from build123d import *

# Parameters (mm, degrees)
F1_DEPTH = 500
F2_R     = 2
F3_R     = 1.5
F4_R     = 1.5


with BuildPart() as f1:
    # F0 (on Front) → F1 (new body)
    with BuildSketch(Plane.XZ):
        Polygon((-12.5, 18.558511), (-22.5, 18.558511), (-22.5, 3.558511), (22.5, 3.558511), (22.5, 18.558511), (12.5, 18.558511), (12.5, 16.058511), (20, 16.058511), (20, 6.058511), (-20, 6.058511), (-20, 16.058511), (-12.5, 16.058511), align=None)
    extrude(amount=F1_DEPTH)

    # F2
    f2_edges = [f1.edges().sort_by_distance(p)[0] for p in [
        (22.5, -250, 18.558511),
        (-22.5, -250, 18.558511),
        (-22.5, -250, 3.558511),
        (22.5, -250, 3.558511),
    ]]
    fillet(f2_edges, radius=F2_R)

    # F3
    f3_edges = [f1.edges().sort_by_distance(p)[0] for p in [
        (20, -250, 16.058511),
        (-20, -250, 16.058511),
    ]]
    fillet(f3_edges, radius=F3_R)

    # F4
    f4_edges = [f1.edges().sort_by_distance(p)[0] for p in [
        (-20, -250, 6.058511),
        (20, -250, 6.058511),
    ]]
    fillet(f4_edges, radius=F4_R)


solid = f1.part
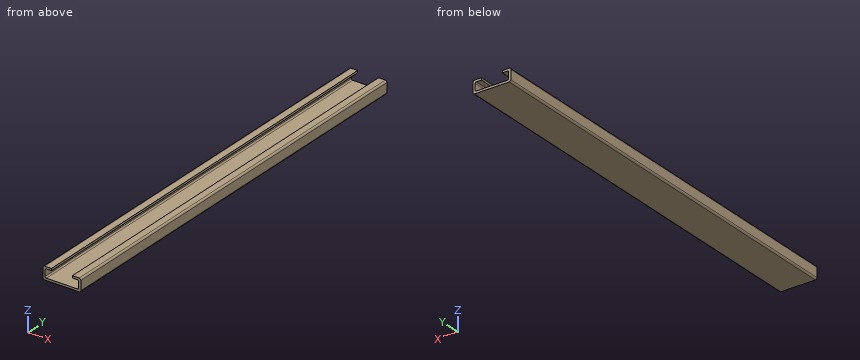
Work out the finished part from the listing and answer in its coordinate system (mm). Give positions to 0.01 mm unless a question says otherwise; leave off trailing zeros. Loops run counter-clockwise (first coordinate to the right, second up) from the corner with the lowest first, then second, coordinate; pieces in that order, holes last. Notation, with made-up numbers: (-32.5, 16) - (-17.5, 16) arc R9 cw to (-17.5, 21) - close; hole circle Ø7 at (32, -30). An arc over 180 degrees is marked (long way). Answer in a Markdown table with one row per item.
(1) Flat-ended cylindrical pins translate along their axes: pin 1 Ø0.8 at (y, z) = (-311.5, 17.5) entering from +X; pin 2 Ø4 at (x, y) = (-3.5, -180.5) entering from +Z; pin 3 Ø2 at (x, z) = (16, 13.5) entering from +Y; pin 4 Ø0.8 at (y, z) = (-248.5, 17) entering from -X. Find the tip coordinate at first contact, or state that the pin passes through.
Results list:
| item | result |
|---|---|
| pin 1 | stops at x = 22.43 |
| pin 2 | stops at z = 6.06 |
| pin 3 | passes through |
| pin 4 | stops at x = -22.5 |
(2) Section A-A (y = -127.5) is taken. Give the vertices of the cut face in (x, z).
Results list:
| item | result |
|---|---|
| outline | (-22.5, 5.56) arc R2 ccw to (-20.5, 3.56) - (20.5, 3.56) arc R2 ccw to (22.5, 5.56) - (22.5, 16.56) arc R2 ccw to (20.5, 18.56) - (12.5, 18.56) - (12.5, 16.06) - (18.5, 16.06) arc R1.5 cw to (20, 14.56) - (20, 7.56) arc R1.5 cw to (18.5, 6.06) - (-18.5, 6.06) arc R1.5 cw to (-20, 7.56) - (-20, 14.56) arc R1.5 cw to (-18.5, 16.06) - (-12.5, 16.06) - (-12.5, 18.56) - (-20.5, 18.56) arc R2 ccw to (-22.5, 16.56) - close |
(3) Consider L1, parallel to X at y = -219, z = 9.5; L2, parallel to Z at x = -18, y = -80.5; L3, parallel to Z at x = -11, y = -145. Determine where each line is inside the solid, lowest interval first. Write a range as [from, to].
Results list:
| item | result |
|---|---|
| L1 | x = [-22.5, -20], [20, 22.5] |
| L2 | z = [3.56, 6.06], [16.06, 18.56] |
| L3 | z = [3.56, 6.06] |
(4) Section C-C (x = 6) is taken. Give the vertices of the cut face in (y, z), and give its area (3 significant figures).
Results list:
| item | result |
|---|---|
| outline | (-500, 3.56) - (0, 3.56) - (0, 6.06) - (-500, 6.06) - close |
| area | 1,250 mm² |
(5) Section B-B (z = 11) is taken. Give the vertices of the cut face in (x, y).
Results list:
| item | result |
|---|---|
| outline | (-22.5, -500) - (-20, -500) - (-20, 0) - (-22.5, 0) - close; (20, -500) - (22.5, -500) - (22.5, 0) - (20, 0) - close |
